Answer from the drawing. Dimensions are ordinates in mm from the lowest x, y and z of the part. A direction names the side the tool comes from. Give positions to 0.01 mm unless a question says otherwise; leave off trailing zeros. Order: outer loops, then holes, each group sorted by start corner. A loop starts at its lowest first (then second) coordinate and runs counter-clockwise, first axis right, second up.
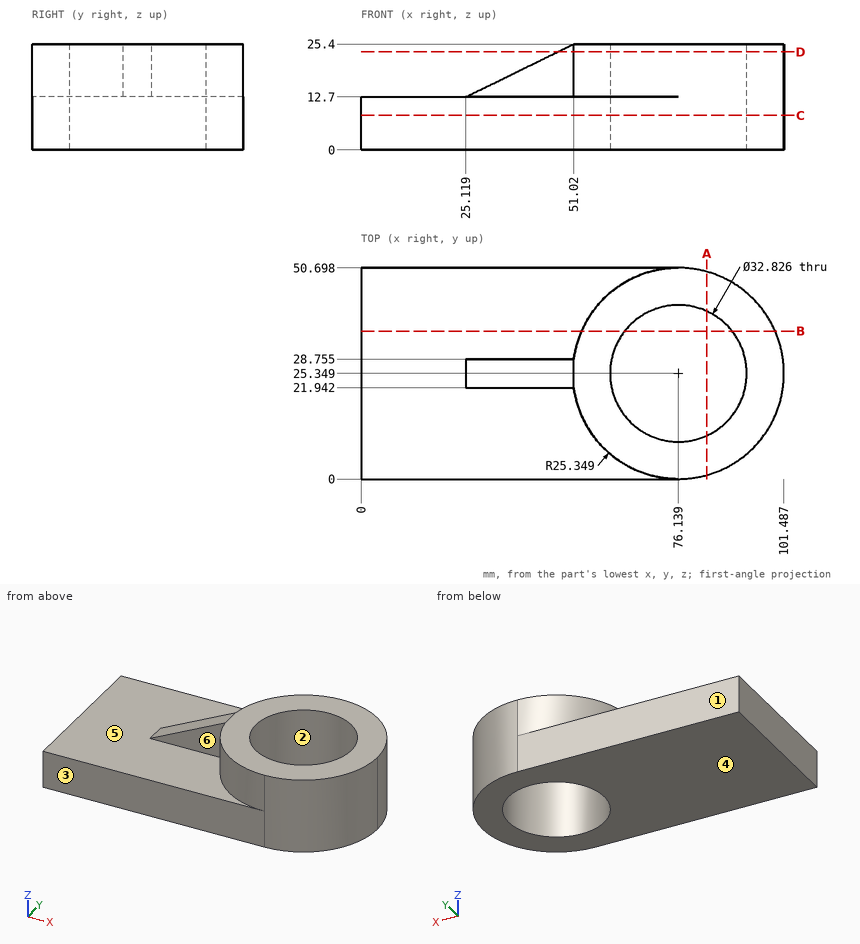
1) The part is cut by section B-B on y = 35.5. Determine the outline of the cut face in (x, z) (1 decimal).
Final values:
outline: (0, 0) - (63.2, 0) - (63.2, 25.4) - (52.9, 25.4) - (52.9, 12.7) - (0, 12.7) - close; (89, 0) - (99.4, 0) - (99.4, 25.4) - (89, 25.4) - close
2) The part is cut by section C-C on z = 8.25. Determine the outline of the cut face in (x, y).
Final values:
outline: (0, 0) - (76.14, 0) arc R25.35 ccw to (101.49, 25.35) arc R25.35 ccw to (76.14, 50.7) - (0, 50.7) - close; hole circle Ø32.83 at (76.14, 25.35)
3) Given pin 1 (3 mm diameter, centred on y = 19.5, z = 20.5, fed in from +X); pin 2 (1.5 mm diameter, centred on y = 26, z = 21, fed in from +X); pin 3 (2 mm diameter, centred on x = 85, z = 19.5, fed in from -Y); pin 4 (10 mm diameter, centred on x = 33, z = 20, fed in from -Y), each flat-ended and moving along its own axis, determine where each tip first touches the part or whether it passes through.
Final values:
pin 1: stops at x = 101.11
pin 2: stops at x = 101.49
pin 3: stops at y = 1.25
pin 4: stops at y = 21.94
4) For a pull along Y with two mould halves and no side action, classify the marked faces 1, 2 and 3 as released by +Y, released by -Y, zero draft, split by the parting line, or undercut.
Final values:
face 1: released by +Y
face 2: undercut
face 3: released by -Y
5) The part is cut by section A-A on x = 83. Determine the outline of the cut face in (y, z), and give its area (3 significant figures).
Final values:
outline: (0.95, 0) - (10.44, 0) - (10.44, 25.4) - (0.95, 25.4) - close; (40.26, 0) - (49.75, 0) - (49.75, 25.4) - (40.26, 25.4) - close
area: 482 mm2
6) A tool of negligible diameter and unlimited length cuts with its end or side. For the marked faces 4, 5 and 6, from which of +Z, -Z, +X, -X, +Y, -Y can it reach the whole face along a straight path? Write none if from no direction.
Final values:
face 4: -Z, +X, -X, +Y, -Y
face 5: +Z, -X
face 6: +Z, -X, -Y
7) Consider L1, parallel to Z at x = 39, y = 8.5; L2, parallel to Y at x = 91, z = 21.5 (1 decimal); L3, parallel to X at y = 40, z = 1 (1 decimal). Determine where each line is inside the solid, lowest interval first.
Final values:
L1: z = 0 to 12.7
L2: y = 4.8 to 18.4, 32.3 to 45.9
L3: x = 0 to 68.7, 83.5 to 96.8
8) The part is cut by section D-D on z = 23.5. Determine the outline of the cut face in (x, y) (1 decimal), and give its area (3 significant figures).
Final values:
outline: (47.1, 21.9) - (51, 21.9) arc R25.3 ccw (long way) to (51, 28.8) - (47.1, 28.8) - close; hole circle Ø32.8 at (76.1, 25.3)
area: 1,200 mm2
